from build123d import *

# Parameters (mm, degrees)
F0_W     = 38.1
F0_H     = 38.1
F1_DEPTH = 0.79375
F2_W     = 38.1
F2_H     = 38.1
F2_W_2   = 34.8996
F2_H_2   = 34.8996
F3_DEPTH = 5.08
F4_W     = 23.4696
F4_H     = 1.27
F4_W_2   = 10.8094774936
F4_W_3   = 18.6369190906
F5_DEPTH = 4.445
F6_R     = 1.27
F7_DEPTH = 0.396875


with BuildPart() as f1:
    # F0 (on Top) → F1 (new body)
    with BuildSketch(Plane.XY):
        with Locations((-39.5794175565, 41.8581605069)):
            Rectangle(F0_W, F0_H)
    extrude(amount=F1_DEPTH)

    # F2 (on face) → F3 (join)
    with BuildSketch(Plane.XY.offset(0.79375)):
        with Locations((-39.5794175565, 41.8581605069)):
            Rectangle(F2_W, F2_H)
        with Locations((-39.5794175565, 41.8581605069)):
            Rectangle(F2_W_2, F2_H_2, mode=Mode.SUBTRACT)
    extrude(amount=F3_DEPTH)

    # F4 (on face) → F5 (join)
    with BuildSketch(Plane.XY.offset(0.79375)):
        Polygon((-51.9492175565, 54.2279605069), (-51.9492175565, 24.4083605069), (-50.6792175565, 24.4083605069), (-50.6792175565, 46.6079605069), (-50.6792175565, 47.8779605069), (-50.6792175565, 52.9579605069), (-50.6792175565, 54.2279605069), align=None)
        Polygon((-50.6792175565, 47.8779605069), (-50.6792175565, 46.6079605069), (-47.1165366471, 46.6079605069), (-45.8465366471, 46.6079605069), (-38.9444175565, 46.6079605069), (-38.9444175565, 47.8779605069), align=None)
        Polygon((-45.8465366471, 46.6079605069), (-47.1165366471, 46.6079605069), (-47.1165366471, 33.9079605069), (-45.8465366471, 33.9079605069), (-45.8465366471, 35.1779605069), align=None)
        with Locations((-38.9444175565, 53.5929605069)):
            Rectangle(F4_W, F4_H)
        with Locations((-27.5343563033, 47.2429605069)):
            Rectangle(F4_W_2, F4_H)
        with Locations((-31.4480771018, 40.8929605069)):
            Rectangle(F4_W_3, F4_H)
        with Locations((-36.5280771018, 34.5429605069)):
            Rectangle(F4_W_3, F4_H)
    extrude(amount=F5_DEPTH)

    # F6 (on face) → F7 (cut)
    with BuildSketch(Plane.XY.offset(0.79375)):
        with Locations((-54.7527819872, 30.2330423146)):
            Circle(F6_R)
        with Locations((-47.7302372456, 28.7605728954)):
            Circle(F6_R)
    extrude(amount=-F7_DEPTH, mode=Mode.SUBTRACT)


solid = f1.part
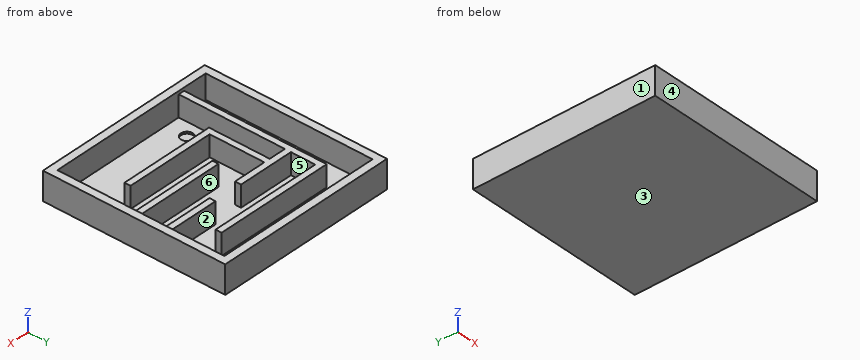
Design review of the part built by this model. Coordinates are the model's own, in mm. Face numbers are marked on the shaded views. A direction names the side the tool comes from. Coordinates: 2 decimals unless noted, no trailing zeros. Order: outer loops, then holes, each group sorted by start corner. A loop starts at its lowest first (then second) coordinate and runs counter-clockwise, first axis right, second up. Notation, with made-up numbers: M -34,-18 L -20,-18 A23 cw -20,14 Z; hole C -3,14 d4. An arc over 180 degrees is marked long. Use a Markdown table: item, result.
(1) Draft analysis for pull direction Y (two halves, no side actions). For the marked faces 3, 4, 5 and 6, state which applies: released by +Y, released by -Y, zero draft, split by the parting line, or undercut.
Worked answers:
| item | result |
|---|---|
| face 3 | zero draft |
| face 4 | released by -Y |
| face 5 | undercut |
| face 6 | undercut |
(2) Add section C-C (y = 29.5). Give the boundary of the cut face in (x, z), then the cut area to 3 significant figures.
Worked answers:
| item | result |
|---|---|
| outline | M -58.63,0 L -20.53,0 L -20.53,5.87 L -22.13,5.87 L -22.13,0.79 L -46.7,0.79 L -46.7,0.4 L -48.76,0.4 L -48.76,0.79 L -50.68,0.79 L -50.68,5.24 L -51.95,5.24 L -51.95,0.79 L -53.72,0.79 L -53.72,0.4 L -55.79,0.4 L -55.79,0.79 L -57.03,0.79 L -57.03,5.87 L -58.63,5.87 Z |
| area | 50.5 mm2 |
(3) For P1, Ø6, axis at x = -32, y = 43, coming from the +Z side; P2, Ø3, axis at x = -35.5, y = 37.5, coming from the +Z side; P3, Ø6, axis at x = -36.5, y = 53.5, coming from the -Z side, all flat-tipped, find the tip position at first contact; note any pin that passes through.
Worked answers:
| item | result |
|---|---|
| P1 | stops at z = 5.24 |
| P2 | stops at z = 0.79 |
| P3 | stops at z = 0 |
(4) Add section D-D (x = -40). Give the boundary of the cut face in (y, z), then the cut area to 3 significant figures.
Worked answers:
| item | result |
|---|---|
| outline | M 22.81,0 L 60.91,0 L 60.91,5.87 L 59.31,5.87 L 59.31,0.79 L 54.23,0.79 L 54.23,5.24 L 52.96,5.24 L 52.96,0.79 L 47.88,0.79 L 47.88,5.24 L 46.61,5.24 L 46.61,0.79 L 41.53,0.79 L 41.53,5.24 L 40.26,5.24 L 40.26,0.79 L 35.18,0.79 L 35.18,5.24 L 33.91,5.24 L 33.91,0.79 L 24.41,0.79 L 24.41,5.87 L 22.81,5.87 Z |
| area | 69.1 mm2 |
(5) Wall thickness on probe 1 along X at (y, z) = (27, 3.85); probe 2 along Y at (x, z) = (-42.5, 3.6); probe 3 along X at (y, z) = (39.5, 5.2): over which ranges is each line inside the solid? List them lowest first.
Worked answers:
| item | result |
|---|---|
| probe 1 | x = -58.63 to -57.03, -51.95 to -50.68, -22.13 to -20.53 |
| probe 2 | y = 22.81 to 24.41, 33.91 to 35.18, 46.61 to 47.88, 52.96 to 54.23, 59.31 to 60.91 |
| probe 3 | x = -58.63 to -57.03, -51.95 to -50.68, -47.12 to -45.85, -22.13 to -20.53 |
(6) Add section B-B (x = -25). Give the boundary of the cut face in (y, z), then the cut area to 3 significant figures.
Worked answers:
| item | result |
|---|---|
| outline | M 22.81,0 L 60.91,0 L 60.91,5.87 L 59.31,5.87 L 59.31,0.79 L 47.88,0.79 L 47.88,5.24 L 46.61,5.24 L 46.61,0.79 L 41.53,0.79 L 41.53,5.24 L 40.26,5.24 L 40.26,0.79 L 24.41,0.79 L 24.41,5.87 L 22.81,5.87 Z |
| area | 57.8 mm2 |
(7) For the marked faces 1 and 2, list the 3-axis set-ups (+Z, -Z, +X, -X, +Y, -Y) from which the entire face can be reached by the end or side of a thin tool; tool diameter is ignored.
Worked answers:
| item | result |
|---|---|
| face 1 | +Z, -Z, -X, +Y, -Y |
| face 2 | +Z |
